Source: three-view drawing plus pictorial views. Frame: mm from the lowest corner of the part. Give positions to 0.01 mm unless a question says otherwise; leave off trailing zeros. Order: outer loops, then holes, each group sorted by start corner. A loop starts at its lowest first (then second) coordinate and runs counter-clockwise, first axis right, second up. Notation, with made-up numbers: (20, -0.5) -> (40, -0.5) arc R3 ccw to (40, 4.5) -> close; hole circle Ø11 at (34, 65). An arc over 180 degrees is marked (long way). Answer in a Markdown table with one row per item.
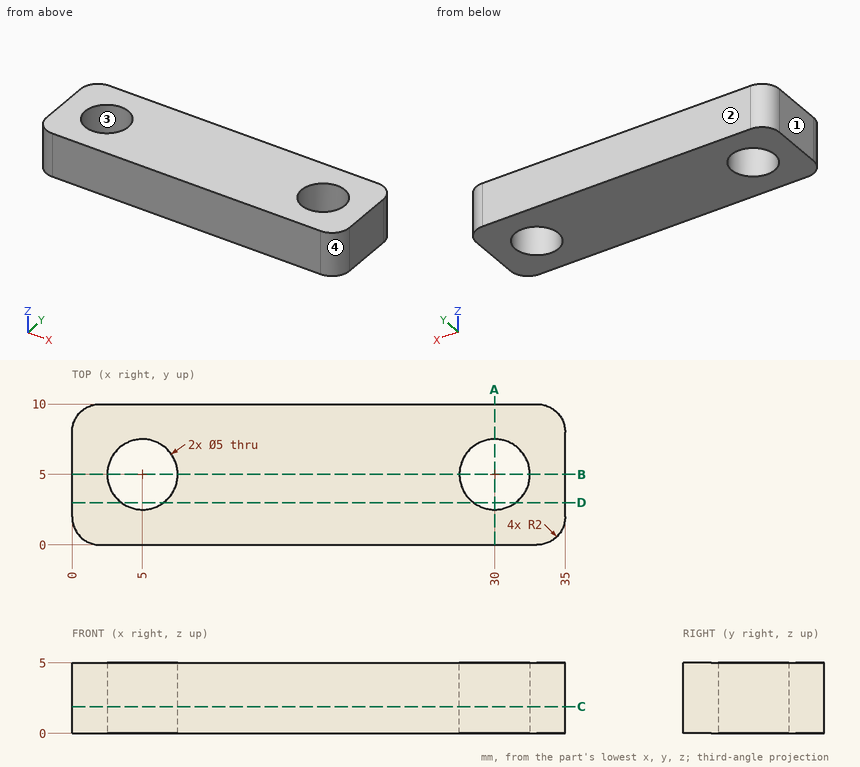
(1) Section query A-A (x = 30). Return the cut outline in (y, z).
A:
| item | result |
|---|---|
| outline | (0, 0) -> (2.5, 0) -> (2.5, 5) -> (0, 5) -> close; (7.5, 0) -> (10, 0) -> (10, 5) -> (7.5, 5) -> close |
(2) Section query D-D (y = 3). Return the cut outline in (x, z).
A:
| item | result |
|---|---|
| outline | (0, 0) -> (3.5, 0) -> (3.5, 5) -> (0, 5) -> close; (6.5, 0) -> (28.5, 0) -> (28.5, 5) -> (6.5, 5) -> close; (31.5, 0) -> (35, 0) -> (35, 5) -> (31.5, 5) -> close |
(3) Pull-direction query (Y, two-part tool) for the marked faces 1, 2, 3 and 4; classes: +Y half, -Y half, draft (parallel to the pull), parting line (faces both ways), or undercut.
A:
| item | result |
|---|---|
| face 1 | draft |
| face 2 | +Y half |
| face 3 | undercut |
| face 4 | -Y half |
(4) Section query C-C (z = 1.9). Return the cut outline in (x, y), plus the area to 3 significant figures.
A:
| item | result |
|---|---|
| outline | (0, 2) arc R2 ccw to (2, 0) -> (33, 0) arc R2 ccw to (35, 2) -> (35, 8) arc R2 ccw to (33, 10) -> (2, 10) arc R2 ccw to (0, 8) -> close; hole circle Ø5 at (5, 5); hole circle Ø5 at (30, 5) |
| area | 307 mm^2 |
(5) Ray query, probe 1 along Y at (x, z) = (5, 3.55); probe 2 along X at (y, z) = (3.25, 4.6); probe 3 along X at (y, z) = (4.25, 2.6). Return the intervals inside material, ascending.
A:
| item | result |
|---|---|
| probe 1 | y = 0 to 2.5, 7.5 to 10 |
| probe 2 | x = 0 to 3.21, 6.79 to 28.21, 31.79 to 35 |
| probe 3 | x = 0 to 2.62, 7.38 to 27.62, 32.38 to 35 |
(6) Section query B-B (y = 5). Return the cut outline in (x, z).
A:
| item | result |
|---|---|
| outline | (0, 0) -> (2.5, 0) -> (2.5, 5) -> (0, 5) -> close; (7.5, 0) -> (27.5, 0) -> (27.5, 5) -> (7.5, 5) -> close; (32.5, 0) -> (35, 0) -> (35, 5) -> (32.5, 5) -> close |
(7) First-contact query: pin 1 Ø4.5 at (x, y) = (5, 5) entering from +Z. Flat tip, straight axial feed; report the tip coordinate or a pass-through.
A:
| item | result |
|---|---|
| pin 1 | passes through |
